Geometry: see drawing. Coordinates: mm, zero at the bounding-box minimum. Coordinates: 2 decimals unless noted, no trailing zeros. Write each loop counter-clockwise with the first axis right and the second up, starting at its lowest first coordinate (ties: lowest second). Pieces come first, ordered by that corner, then holes.
1) Section query D-D (x = 26). Output: boundary loops of the cut face in (y, z).
2) Section query A-A (x = 9.75). Output: boundary loops of the cut face in (y, z), then the cut area to 3 significant figures.
3) Section query C-C (y = 12). Output: boundary loops of the cut face in (x, z).
4) Draft query along X for the marked faces 1 and 2. Return one class per face: pulls with the +X half, pulls with the -X half, needs draft (parallel to the pull), parting line crosses it, or undercut.
5) Pin query (flat end, axial travel): pin 1 Ø0.6 at (y, z) = (28, 2) entering from -X; pin 2 Ø1 at (x, y) = (23.5, 41) entering from +Z; pin 3 Ø0.6 at (x, z) = (45, 2) entering from -Y; pin 4 Ø3 at (x, y) = (29, 8) entering from -Z. Return the tip coordinate at first contact, or that it passes through.
6) Section query B-B (z = 4.65). Output: boundary loops of the cut face in (x, y), then the cut area to 3 significant figures.
7) Line query: L1, parallel to Y at x = 42.25, z = 0.85; L2, parallel to Y at x = 43.5, z = 2.8; L3, parallel to X at y = 7, z = 3.35. Output: solid intervals per line, ascending.
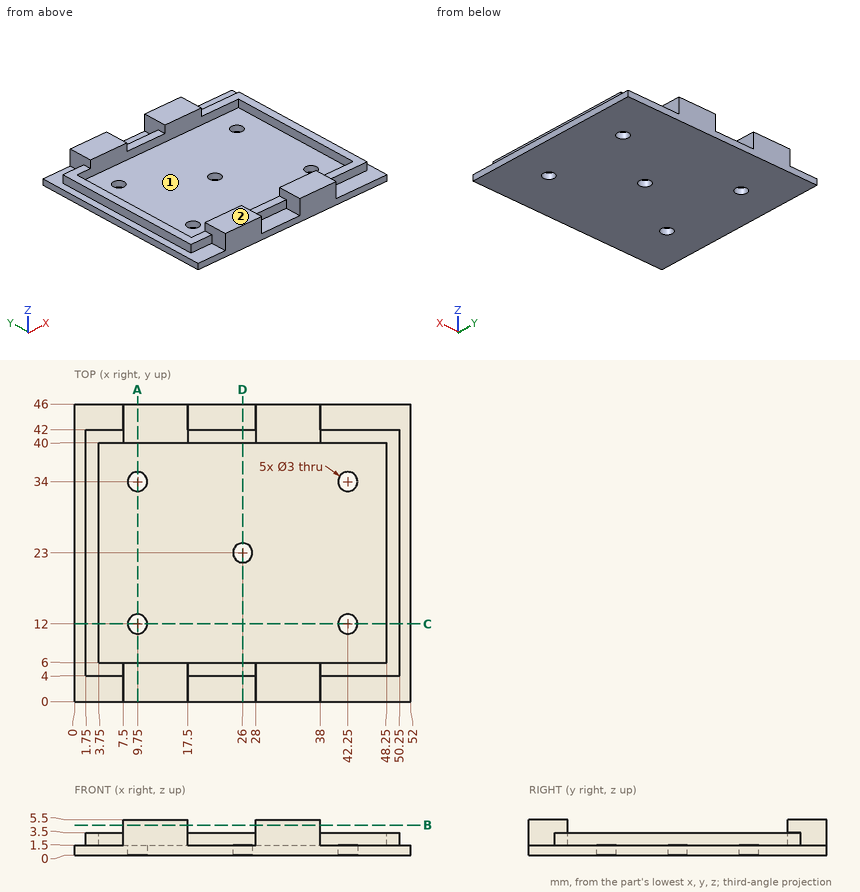
Answer:
1. outline: (0, 0) - (21.5, 0) - (21.5, 1.5) - (6, 1.5) - (6, 3.5) - (4, 3.5) - (4, 1.5) - (0, 1.5) - close; (24.5, 0) - (46, 0) - (46, 1.5) - (42, 1.5) - (42, 3.5) - (40, 3.5) - (40, 1.5) - (24.5, 1.5) - close
2. outline: (0, 0) - (10.5, 0) - (10.5, 1.5) - (6, 1.5) - (6, 5.5) - (0, 5.5) - close; (13.5, 0) - (32.5, 0) - (32.5, 1.5) - (13.5, 1.5) - close; (35.5, 0) - (46, 0) - (46, 5.5) - (40, 5.5) - (40, 1.5) - (35.5, 1.5) - close
2. area: 108 mm2
3. outline: (0, 0) - (8.25, 0) - (8.25, 1.5) - (3.75, 1.5) - (3.75, 3.5) - (1.75, 3.5) - (1.75, 1.5) - (0, 1.5) - close; (11.25, 0) - (40.75, 0) - (40.75, 1.5) - (11.25, 1.5) - close; (43.75, 0) - (52, 0) - (52, 1.5) - (50.25, 1.5) - (50.25, 3.5) - (48.25, 3.5) - (48.25, 1.5) - (43.75, 1.5) - close
4. face 1: undercut
4. face 2: needs draft
5. pin 1: stops at x = 1.75
5. pin 2: stops at z = 3.5
5. pin 3: stops at y = 4
5. pin 4: stops at z = 0
6. outline: (7.5, 0) - (17.5, 0) - (17.5, 6) - (7.5, 6) - close; (7.5, 40) - (17.5, 40) - (17.5, 46) - (7.5, 46) - close; (28, 0) - (38, 0) - (38, 6) - (28, 6) - close; (28, 40) - (38, 40) - (38, 46) - (28, 46) - close
6. area: 240 mm2
7. L1: y = 0 to 10.5, 13.5 to 32.5, 35.5 to 46
7. L2: y = 4 to 6, 40 to 42
7. L3: x = 1.75 to 3.75, 48.25 to 50.25
